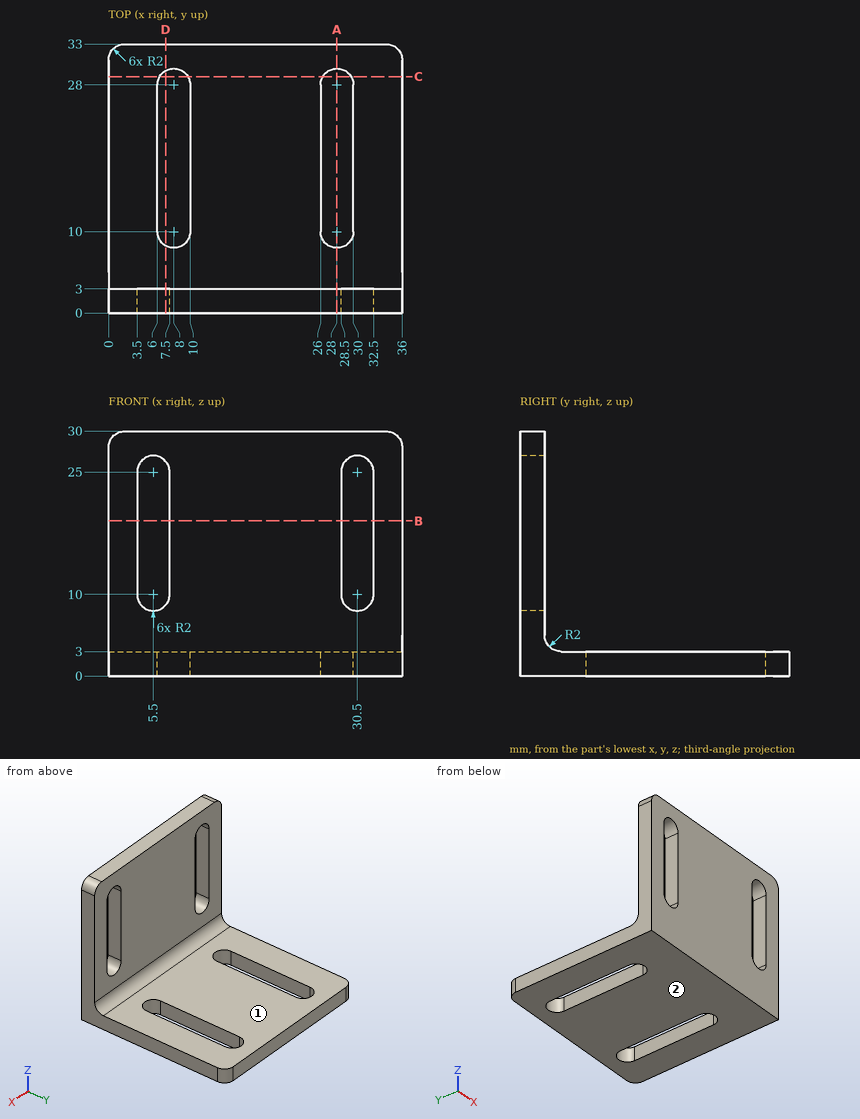
Here's the drawing with two shaded views (mm, measured from the low corner). I have some questions. A direction names the side the tool comes from. Round coordinates to 2 decimals unless told otherwise and drop trailing zeros. Loops run counter-clockwise (first coordinate to the right, second up) from the corner with the lowest first, then second, coordinate; pieces in that order, holes last. Notation, with made-up numbers: (-9, -4) - (38, -4) arc R30 cw to (38, 22) - close; hole circle Ø10 at (74.25, 12.5). An arc over 180 degrees is marked (long way). Use CSV: the item, a comma, the result in double quotes. Start each with the question number.
1) If we section it at B-B on z = 19: Write out the boundary of the cut face in (x, y), plus the area to 3 significant figures.
2) If we section it at D-D on x = 7: Write out the boundary of the cut face in (y, z), plus the area to 3 significant figures.
3) For pin 1 Ø2.5 at (y, z) = (1.5, 16) entering from -X; pin 2 Ø3 at (x, y) = (30.5, 27.5) entering from +Z; pin 3 Ø12.5 at (x, z) = (22.5, 19) entering from +Y, each with a flat end and sliding along its axis, tell me the tip position at first contact or that it passes through.
4) Please list where these lines run through material, in increasing order: probe 1 along X at (y, z) = (11.5, 2.25); probe 2 along Y at (x, z) = (34, 14.5). Write a range as [from, to].
5) If we section it at C-C on y = 29: Write out the boundary of the cut face in (x, z), plus the area to 3 significant figures.
6) For the marked faces 1 and 2, which set-ups out of +Z, -Z, +X, -X, +Y, -Y let a thin tool reach every point of the face, with its end or its side?
7) If we section it at A-A on x = 28: Write out the boundary of the cut face in (y, z).
Geometry results:
1,outline,"(0, 0) - (3.5, 0) - (3.5, 3) - (0, 3) - close; (7.5, 0) - (28.5, 0) - (28.5, 3) - (7.5, 3) - close; (32.5, 0) - (36, 0) - (36, 3) - (32.5, 3) - close"
1,area,"84.0 mm2"
2,outline,"(0, 0) - (8.27, 0) - (8.27, 3) - (5, 3) arc R2 cw to (3, 5) - (3, 8.68) - (0, 8.68) - close; (0, 26.32) - (3, 26.32) - (3, 30) - (0, 30) - close; (29.73, 0) - (33, 0) - (33, 3) - (29.73, 3) - close"
2,area,"63.5 mm2"
3,pin 1,"stops at x = 0"
3,pin 2,"stops at z = 3"
3,pin 3,"stops at y = 3"
4,probe 1,"x = [0, 6], [10, 26], [30, 36]"
4,probe 2,"y = [0, 3]"
5,outline,"(0, 0) - (6.27, 0) - (6.27, 3) - (0, 3) - close; (9.73, 0) - (26.27, 0) - (26.27, 3) - (9.73, 3) - close; (29.73, 0) - (36, 0) - (36, 3) - (29.73, 3) - close"
5,area,"87.2 mm2"
6,face 1,"+Z, +X, -X, +Y"
6,face 2,"-Z, +X, -X, +Y, -Y"
7,outline,"(0, 0) - (8, 0) - (8, 3) - (5, 3) arc R2 cw to (3, 5) - (3, 30) - (0, 30) - close; (30, 0) - (33, 0) - (33, 3) - (30, 3) - close"
